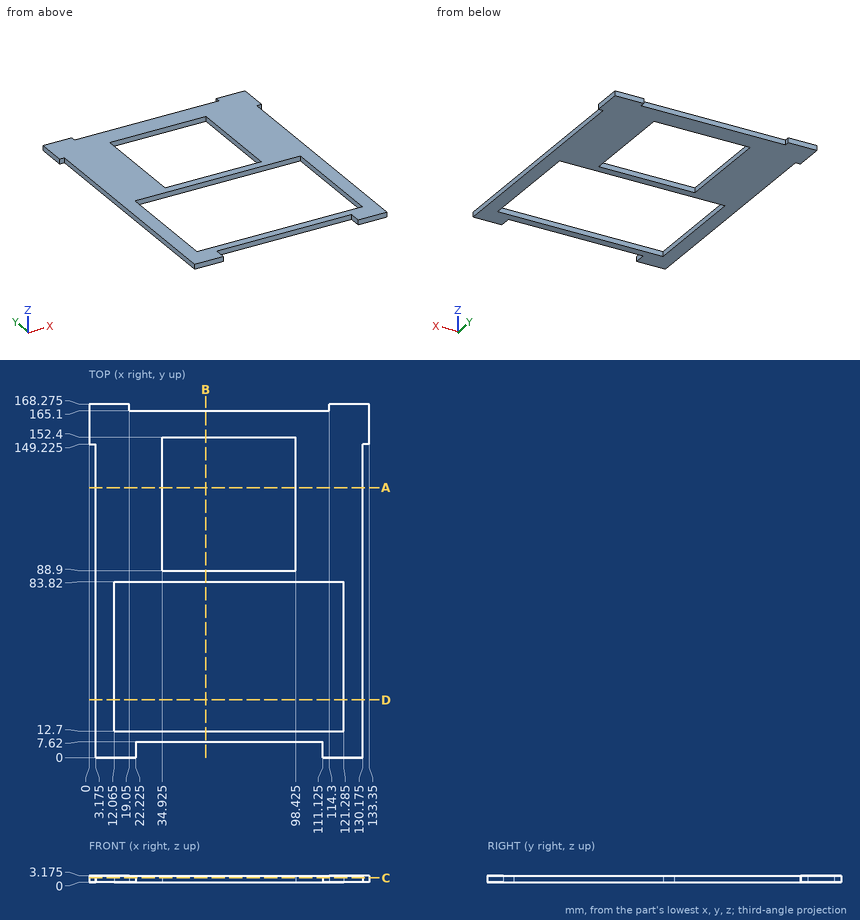
The drawing under review shows one solid part. Ordinate dimensions are in mm from its lowest x, y, z. Round coordinates to 2 decimals unless told otherwise and drop trailing zeros. Loops run counter-clockwise (first coordinate to the right, second up) from the corner with the lowest first, then second, coordinate; pieces in that order, holes last. Notation, with made-up numbers: (44, 54) - (90, 54) arc R24 ccw to (90, 77) - close; hole circle Ø7 at (-37.75, -24.5). An arc over 180 degrees is marked (long way). Put each result on its own line as item: value. Start each with the question number.
1. Consider section A-A on y = 128.5. State the section outline as (x, z) points (3 decimals).
2. Consider section B-B on x = 55.5. State the section outline as (y, z) points (3 decimals).
3. For probe 1 along Y at (x, z) = (59.5, 2.4); probe 2 along X at (y, z) = (132, 0.25) (3 decimals); probe 3 along Y at (x, z) = (19, 2) (3 decimals), list the stretches that pass through material, from the lowest coordinate up. Write a range as [from, to].
4. Consider section C-C on z = 2.15. State the section outline as (x, y) points (3 decimals).
5. Consider section D-D on y = 27.5. State the section outline as (x, z) points (3 decimals), plus the area to 3 significant figures.
6. Insertion check: P1, Ø1.6, axis at x = 50.5, z = 1.5, coming from the +Y side; P2, Ø1.6, axis at x = 1, z = 1.5, coming from the -Y side (3 decimals); P3, Ø1.5, axis at y = 60, z = 2.5, coming from the +X side (3 decimals). Each pin has a flat end and moves straight along its axis. Give the tip position at first contact, or say it passes through.
Result sheet:
1. outline: (3.175, 0) - (34.925, 0) - (34.925, 3.175) - (3.175, 3.175) - close; (98.425, 0) - (130.175, 0) - (130.175, 3.175) - (98.425, 3.175) - close
2. outline: (7.62, 0) - (12.7, 0) - (12.7, 3.175) - (7.62, 3.175) - close; (83.82, 0) - (88.9, 0) - (88.9, 3.175) - (83.82, 3.175) - close; (152.4, 0) - (165.1, 0) - (165.1, 3.175) - (152.4, 3.175) - close
3. probe 1: [7.62, 12.7], [83.82, 88.9], [152.4, 165.1]
3. probe 2: [3.175, 34.925], [98.425, 130.175]
3. probe 3: [0, 12.7], [83.82, 168.275]
4. outline: (0, 149.225) - (3.175, 149.225) - (3.175, 0) - (22.225, 0) - (22.225, 7.62) - (111.125, 7.62) - (111.125, 0) - (130.175, 0) - (130.175, 149.225) - (133.35, 149.225) - (133.35, 168.275) - (114.3, 168.275) - (114.3, 165.1) - (19.05, 165.1) - (19.05, 168.275) - (0, 168.275) - close; hole (12.065, 12.7) - (121.285, 12.7) - (121.285, 83.82) - (12.065, 83.82) - close; hole (34.925, 88.9) - (98.425, 88.9) - (98.425, 152.4) - (34.925, 152.4) - close
5. outline: (3.175, 0) - (12.065, 0) - (12.065, 3.175) - (3.175, 3.175) - close; (121.285, 0) - (130.175, 0) - (130.175, 3.175) - (121.285, 3.175) - close
5. area: 56.5 mm^2
6. P1: y = 165.1
6. P2: y = 149.225
6. P3: x = 130.175
